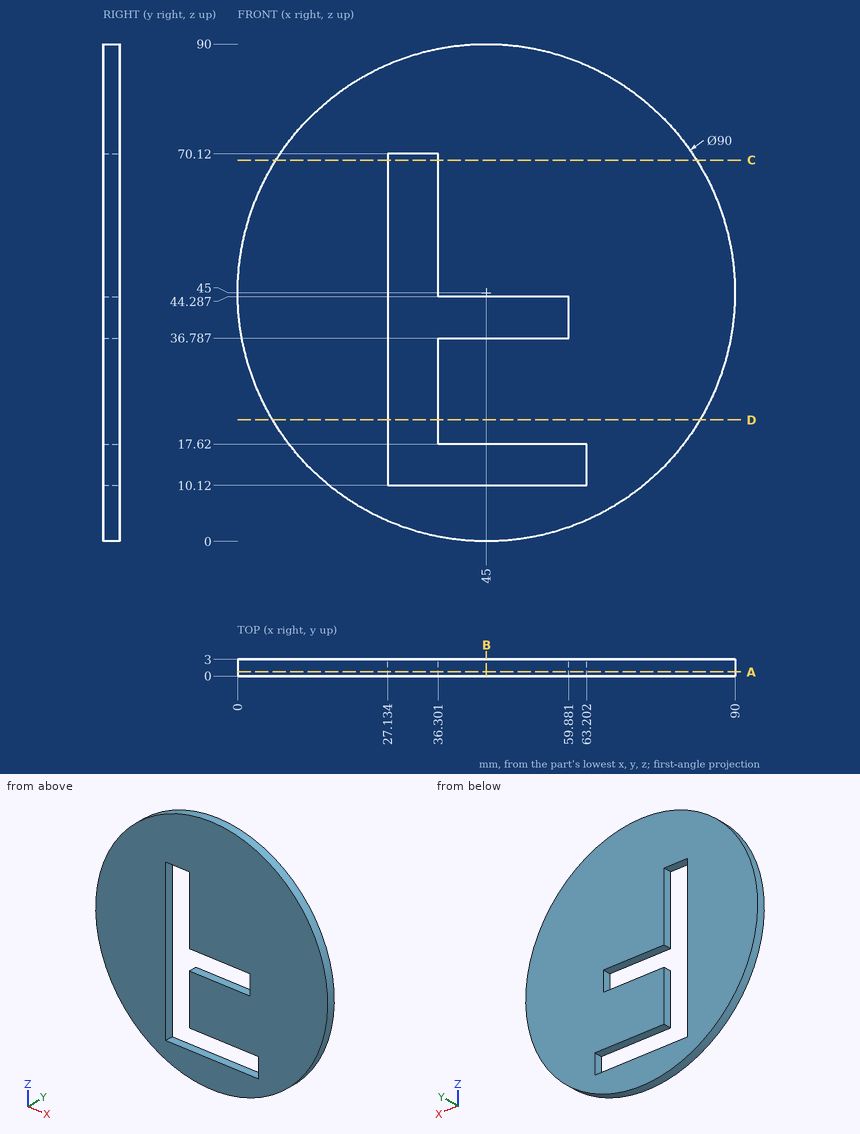
Check sheet for the drawn part. Datum: minimum x, y, z corner. Units: mm. Give positions to 0.01 mm unless a question says otherwise; leave off trailing zeros. Order: outer loops, then holes, each group sorted by start corner. A loop starts at its lowest first (then second) coordinate and runs counter-clockwise, first axis right, second up. Notation, with made-up numbers: (-35.5, 19) -> (-4.5, 19) arc R32 cw to (-4.5, 50) -> close; hole circle Ø7 at (31.25, 69). An arc over 180 degrees is marked (long way). One line per item, written item: value.
(1) Sectioned sample at D-D on z = 22. Record the cut outline in (x, y).
Final values:
outline: (6.32, 0) -> (27.13, 0) -> (27.13, 3) -> (6.32, 3) -> close; (36.3, 0) -> (83.68, 0) -> (83.68, 3) -> (36.3, 3) -> close
(2) Scan lines: line 1 along Z through (x, y) = (45.5, 1.55); line 2 along Z through (x, y) = (39.5, 0.7); line 3 along X through (y, z) = (0.8, 13.5) (1 decimal). Record each from-to range of solid material in increasing order. Write a range as [from, to].
Final values:
line 1: [0, 10.12], [17.62, 36.79], [44.29, 90]
line 2: [0.34, 10.12], [17.62, 36.79], [44.29, 89.66]
line 3: [12.9, 27.1], [63.2, 77.1]
(3) Sectioned sample at C-C on z = 69. Record the cut outline in (x, y) (1 decimal).
Final values:
outline: (6.9, 0) -> (27.1, 0) -> (27.1, 3) -> (6.9, 3) -> close; (36.3, 0) -> (83.1, 0) -> (83.1, 3) -> (36.3, 3) -> close
(4) Sectioned sample at A-A on y = 0.75. Record the cut outline in (x, z).
Final values:
outline: circle Ø90 at (45, 45); hole (27.13, 10.12) -> (63.2, 10.12) -> (63.2, 17.62) -> (36.3, 17.62) -> (36.3, 36.79) -> (59.88, 36.79) -> (59.88, 44.29) -> (36.3, 44.29) -> (36.3, 70.12) -> (27.13, 70.12) -> close
(5) Gauge pin test, flat ends, axial feed: pin 1 (0.9 mm diameter, centred on x = 53, y = 1.5, fed in from -Z); pin 2 (0.9 mm diameter, centred on x = 50.5, y = 1, fed in from +Z); pin 3 (1.5 mm diameter, centred on x = 32, y = 1, fed in from -Z); pin 4 (12 mm diameter, centred on x = 32, z = 81, fed in from -Y). Record the tip position at first contact, or that the pin passes through.
Final values:
pin 1: z = 0.64
pin 2: z = 89.72
pin 3: z = 1.7
pin 4: y = 0
(6) Sectioned sample at B-B on x = 45. Record the cut outline in (y, z).
Final values:
outline: (0, 0) -> (3, 0) -> (3, 10.12) -> (0, 10.12) -> close; (0, 17.62) -> (3, 17.62) -> (3, 36.79) -> (0, 36.79) -> close; (0, 44.29) -> (3, 44.29) -> (3, 90) -> (0, 90) -> close
